Study the drawing (mm; zero at the part's minimum x, y, z) and answer. Coordinates: 2 decimals unless noted, no trailing zeros. Order: outer loops, then holes, each group sorted by start corner. A loop starts at its lowest first (then second) coordinate and runs counter-clockwise, first axis right, second up. Notation, with made-up numbers: M -28,33.25 L 1,33.25 A10 cw 1,37.25 Z; hole C 25,89 d5. An arc over 180 degrees is marked long. Use a Markdown table: item, result. Add a question column.
1) Each of these flat-tipped pins is pushed along its axis until it touches: pin 1 Ø4.5 at (x, y) = (96.5, 3.5) entering from +Z; pin 2 Ø1.2 at (x, z) = (2.5, 1.5) entering from +Y; pin 3 Ø1.6 at (y, z) = (59.5, 1.5) entering from -X; pin 4 Ø0.8 at (x, z) = (97.5, 1.5) entering from -Y. Where does it stop, or does it pass through?
2) Find the intervals of material crossed by probe 1 along X at (y, z) = (58.5, 1.9); probe 2 along Y at (x, z) = (96.5, 2.15); probe 3 along X at (y, z) = (13.5, 0.5), in increasing order. Write a range as [from, to].
3) Find section B-B on y = 29. Write down the section's boundary in (x, z), plus the area to 3 significant figures.
4) Find section A-A on x = 40. Write down the section's boundary in (y, z), plus the area to 3 significant figures.
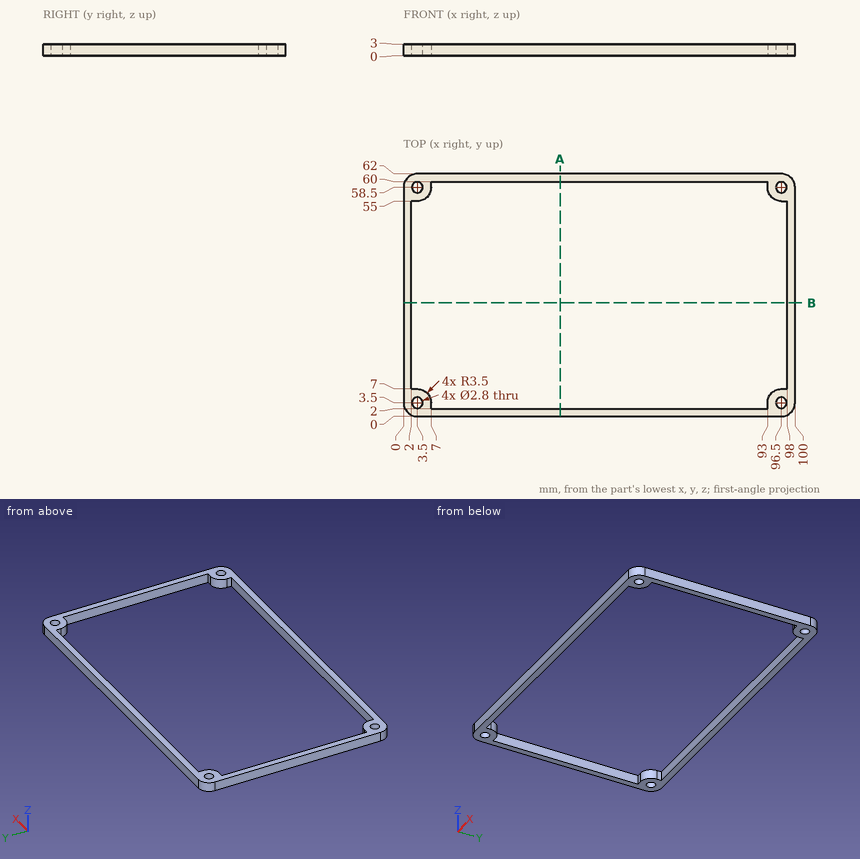
Check result:
| question | item | result |
|---|---|---|
| 1 | pin 1 | stops at z = 3 |
| 1 | pin 2 | stops at y = 61.98 |
| 1 | pin 3 | stops at x = 0.01 |
| 1 | pin 4 | stops at y = 0.05 |
| 2 | probe 1 | x = [0, 2.1], [4.9, 7], [93, 95.1], [97.9, 100] |
| 2 | probe 2 | y = [0, 2.1], [4.9, 7], [55, 57.1], [59.9, 62] |
| 2 | probe 3 | x = [0, 2], [98, 100] |
| 3 | outline | M 0,0 L 2,0 L 2,3 L 0,3 Z; M 98,0 L 100,0 L 100,3 L 98,3 Z |
| 3 | area | 12.0 mm2 |
| 4 | outline | M 0,0 L 2,0 L 2,3 L 0,3 Z; M 60,0 L 62,0 L 62,3 L 60,3 Z |
| 4 | area | 12.0 mm2 |
